from build123d import *

# Parameters (mm, degrees)
F1_DEPTH  = 10.1854
F4_DEPTH  = 34.2265
F6_DEPTH  = 36.5262
F7_R      = 1.5875
F9_DEPTH  = 6.35
F10_R     = 1.190625
F11_DEPTH = 1.5885


with BuildPart() as f1:
    # F0 (on Top) → F1 (new body)
    with BuildSketch(Plane.XY):
        with BuildLine():
            Line((33.3248, -9.12495), (-33.3248, -9.12495))
            ThreePointArc((-33.3248, -9.12495), (-30.652164023, -15.577264023), (-24.19985, -18.2499))
            Line((-24.19985, -18.2499), (24.19985, -18.2499))
            ThreePointArc((24.19985, -18.2499), (30.652164023, -15.577264023), (33.3248, -9.12495))
        make_face()
        with BuildLine():
            Line((24.19985, 0), (0, 0))
            Line((0, 0), (-24.19985, 0))
            ThreePointArc((-24.19985, 0), (-30.652164023, -2.672635977), (-33.3248, -9.12495))
            Line((-33.3248, -9.12495), (33.3248, -9.12495))
            ThreePointArc((33.3248, -9.12495), (30.652164023, -2.672635977), (24.19985, 0))
        make_face()
    extrude(amount=F1_DEPTH)

    # F2: F1 across plane


with BuildPart() as f1_1:
    add(f1.part)
    add(f1.part.mirror(Plane.XZ))

    # F3 (on Right) → F4 (join, symmetric)
    with BuildSketch(Plane.YZ):
        Polygon((-16.6751, 0), (-18.2626, 0), (-18.2626, -3.175), (0, -3.175), (0, -1.5875), (-16.6751, -1.5875), align=None)
        Polygon((0, -1.5875), (0, -3.175), (18.2626, -3.175), (18.2626, 0), (16.6751, 0), (16.6751, -1.5875), align=None)
    extrude(amount=F4_DEPTH, both=True)

    # F5 (on face) → F6 (cut, through all)
    with BuildSketch(Plane.XZ.offset(18.2626)):
        Polygon((-34.2265, 0), (-34.2265, -1.5875), (-31.6865, -1.5875), (-31.6865, -0.635), (-31.0515, 0), align=None)
        Polygon((34.2265, 0), (31.0515, 0), (31.6865, -0.635), (31.6865, -1.5875), (34.2265, -1.5875), align=None)
    extrude(amount=-F6_DEPTH, mode=Mode.SUBTRACT)

    # F7
    f7_edges = [f1_1.edges().sort_by_distance(p)[0] for p in [
        (-34.2265, -18.2626, -2.38125),
        (-34.2265, 18.2626, -2.38125),
        (34.2265, -18.2626, -2.38125),
        (34.2265, 18.2626, -2.38125),
    ]]
    fillet(f7_edges, radius=F7_R)

    # F8 (on Front) → F9 (join, symmetric)
    with BuildSketch(Plane.XZ):
        Polygon((-32.639, -3.175), (-34.2265, -3.175), (-34.2265, -15.5575), (-42.1005, -15.5575), (-42.1005, -17.145), (-32.639, -17.145), align=None)
        Polygon((32.639, -3.175), (32.639, -17.145), (42.1005, -17.145), (42.1005, -15.5575), (34.2265, -15.5575), (34.2265, -3.175), align=None)
    extrude(amount=F9_DEPTH, both=True)

    # F10 (on face) → F11 (cut, through all)
    with BuildSketch(Plane.XY.offset(-15.5575)):
        with BuildLine():
            ThreePointArc((-39.354125, 0), (-38.1635, -1.190625), (-36.972875, 0))
            Line((-36.972875, 0), (-38.1635, 0))
            Line((-38.1635, 0), (-39.354125, 0))
        make_face()
        with BuildLine():
            Line((-38.1635, 0), (-36.972875, 0))
            ThreePointArc((-36.972875, 0), (-38.1635, 1.190625), (-39.354125, 0))
            Line((-39.354125, 0), (-38.1635, 0))
        make_face()
        with Locations((38.1635, 0)):
            Circle(F10_R)
    extrude(amount=-F11_DEPTH, mode=Mode.SUBTRACT)


solid = f1_1.part
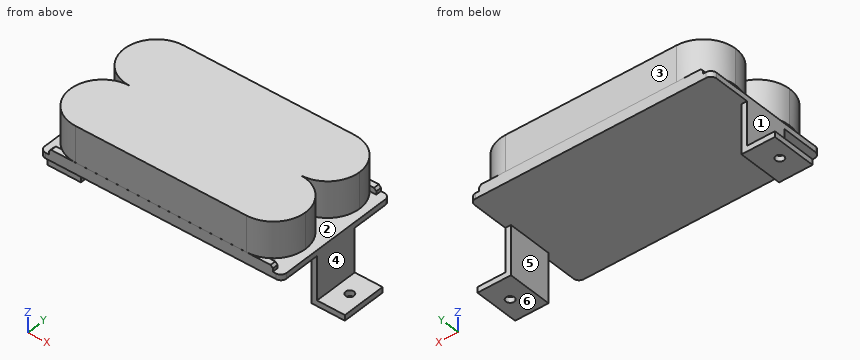
The listing builds one solid part. Answer for the finished solid, in the listing's coordinates (mm). Face numbers are marked on the shaded views. A direction names the side the tool comes from. Coordinates: 2 decimals unless noted, no trailing zeros. Loops run counter-clockwise (first coordinate to the right, second up) from the corner with the lowest first, then second, coordinate; pieces in that order, holes last. Notation, with made-up numbers: (41, -9.5) -> (47, -9.5) arc R14 cw to (47, 14.5) -> close; hole circle Ø10 at (25.25, 8.5). An arc over 180 degrees is marked (long way). Answer in a Markdown table with one row per item. Add a question column.
1. For the marked faces 4, 5 and 6, determine the directions among +Z, -Z, +X, -X, +Y, -Y from which every point of the face is accessible in a straight line to the end or side of a thin tool.
2. The part is cut by section D-D, the plane z = 4.75. Write down the section's boundary in (x, y).
3. Consider line 1 (Z direction, x = -12, y = 11) (1 decimal); line 2 (Y direction, x = 21.5, z = -0.5); line 3 (Y direction, x = 1.5, z = 5.75). Determine where each line is inside the solid, lowest interval first. Write a range as [from, to].
4. The part is cut by section A-A, the plane z = -12. Write down the section's boundary in (x, y), then the cut area to 3 significant figures.
5. Determine the mould class of the marked faces 1, 2 and 3 for opening direction Y: +Y half, -Y half, draft (parallel to the pull), parting line (faces both ways), or undercut.
6. The part is cut by section B-B, the plane y = -5. Write down the section's boundary in (x, z) (1 decimal).
7. Flat-ended cylindrical pins translate along their axes: P1, Ø7.5, axis at x = -37.5, z = -10, coming from the +Y side; P2, Ø5, axis at x = 14, y = 2.5, coming from the -Z side (3 decimals); P3, Ø10, axis at y = 6.5, z = 7, coming from the +X side. Find the tip coordinate at first contact, or state that the pin passes through.
Answer below:
| question | item | result |
|---|---|---|
| 1 | face 4 | +Z, +X, +Y, -Y |
| 1 | face 5 | -Z, +Y, -Y |
| 1 | face 6 | -Z, +X, -X, +Y, -Y |
| 2 | outline | (-24.2, -18.25) -> (24.2, -18.25) arc R9.12 ccw to (24.2, 0) arc R9.12 ccw to (24.2, 18.25) -> (-24.2, 18.25) arc R9.12 ccw to (-24.2, 0) arc R9.12 ccw to start |
| 3 | line 1 | [-3.2, -1.6], [0, 10.2] |
| 3 | line 2 | [-18.26, -16.68], [16.68, 18.26] |
| 3 | line 3 | [-18.25, 18.25] |
| 4 | outline | (-34.23, -6.35) -> (-32.64, -6.35) -> (-32.64, 6.35) -> (-34.23, 6.35) -> close; (32.64, -6.35) -> (34.23, -6.35) -> (34.23, 6.35) -> (32.64, 6.35) -> close |
| 4 | area | 40.3 mm2 |
| 5 | face 1 | draft |
| 5 | face 2 | undercut |
| 5 | face 3 | +Y half |
| 6 | outline | (-42.1, -17.1) -> (-32.6, -17.1) -> (-32.6, -3.2) -> (32.6, -3.2) -> (32.6, -17.1) -> (42.1, -17.1) -> (42.1, -15.6) -> (34.2, -15.6) -> (34.2, -1.6) -> (-34.2, -1.6) -> (-34.2, -15.6) -> (-42.1, -15.6) -> close; (-32.3, 0) -> (32.3, 0) -> (32.3, 10.2) -> (-32.3, 10.2) -> close |
| 7 | P1 | y = 6.35 |
| 7 | P2 | z = -3.175 |
| 7 | P3 | x = 33.32 |
